from build123d import *

# Parameters (mm, degrees)
SKETCH1_W                = 45.72
SKETCH1_H                = 119.38
BOSS_EXTRUDE1_DEPTH      = 1.27
BOSS_EXTRUDE1_DEPTH_BACK = 7.636822689
SKETCH2_W                = 39.878
SKETCH2_H                = 113.538
SKETCH2_W_2              = 38.862
SKETCH2_H_2              = 112.522
BOSS_EXTRUDE2_DEPTH      = 2.54
SKETCH4_R                = 3.175
CUT_EXTRUDE1_DEPTH       = 12.446822689
SKETCH12_W               = 39.37
SKETCH12_H               = 112.522
CUT_EXTRUDE3_DEPTH       = 7.112


with BuildPart() as part:
    # Sketch1 → Boss-Extrude1 (new body, two sides)
    with BuildSketch(Plane.XY) as boss_extrude1_sk:
        with Locations((-64.545156171, 15.983606897)):
            Rectangle(SKETCH1_W, SKETCH1_H)
    extrude(amount=BOSS_EXTRUDE1_DEPTH)
    extrude(boss_extrude1_sk.sketch, amount=-BOSS_EXTRUDE1_DEPTH_BACK)

    # Sketch2 → Boss-Extrude2 (add)
    with BuildSketch(Plane.XY.offset(1.27)):
        with Locations((-64.545156171, 15.983606897)):
            Rectangle(SKETCH2_W, SKETCH2_H)
        with Locations((-64.545156171, 15.983606897)):
            Rectangle(SKETCH2_W_2, SKETCH2_H_2, mode=Mode.SUBTRACT)
    extrude(amount=BOSS_EXTRUDE2_DEPTH)

    # Sketch4 → Cut-Extrude1 (cut, through all)
    with BuildSketch(Plane(origin=(0, 0, -7.636822689), x_dir=(-1, 0, 0), z_dir=(0, 0, -1))):
        with Locations((75.500176171, 1.792626897)):
            Circle(SKETCH4_R)
    extrude(amount=-CUT_EXTRUDE1_DEPTH, mode=Mode.SUBTRACT)

    # Sketch12 → Cut-Extrude3 (cut)
    with BuildSketch(Plane.XY.offset(1.27)):
        with Locations((-64.545156171, 16.237606897)):
            Rectangle(SKETCH12_W, SKETCH12_H)
    extrude(amount=-CUT_EXTRUDE3_DEPTH, mode=Mode.SUBTRACT)


solid = part.part
Model file for the job. Use its own axes, mm. A direction names the side the tool comes from. Coordinates: 2 decimals unless noted, no trailing zeros. Order: outer loops, then holes, each group sorted by start corner. A loop starts at its lowest first (then second) coordinate and runs counter-clockwise, first axis right, second up. Notation, with made-up numbers: (29, -12.5) -> (51, -12.5) arc R22 ccw to (51, -6.5) -> close; hole circle Ø8 at (5.25, 53). An arc over 180 degrees is marked (long way). Return JSON: item names as keys, results as strings. Group by question number.
Item 1: Flat gauge pins, fed straight in: P1, Ø1.3, axis at y = 5.5, z = 3, coming from the +X side; P2, Ø12, axis at x = -71, y = 16, coming from the +Z side; P3, Ø3, axis at x = -61, z = 3, coming from the -Y side. Where does each tip first touch, or does it go through?
Item 2: Pull direction X, two halves, no side cores. Call faces 1 (the flat face through (-85, 21, 1.27)), 2 (the flat face through (-44.86, 15, -2)), 3 (the flat face through (-87.405, 15, -3)): pulls with the +X half, pulls with the -X half, needs draft (parallel to the pull), parting line crosses it, or undercut.
Item 3: Tool access for faces 4 (the flat face through (-65, 72.245, 3)), 5 (the flat face through (-65, -40.785, 3)), 6 (the flat face through (-65, 72.753, 3)), 7 (the flat face through (-84.23, 15, -2)): list every direction of +Z, -Z, +X, -X, +Y, -Y with a clear straight run to the whole face (end or side of a thin tool).
Item 4: Saw through at C-C on y = 24. Write the cut outline in (x, z), then the cut area to 3 significant figures.
Item 5: Wall check: line 1 along X through (y, z) = (-15, 3.75); line 2 along X through (y, z) = (-8, 0); line 3 along Y through (x, z) = (-74, -2.5). Give the ranges that are in metal, low to high. Write a range as [from, to].
Item 6: Saw through at A-A on z = 0. Write the cut outline in (x, y), then the cut area to 3 significant figures.
Item 7: Saw through at D-D on x = -66. Write the cut outline in (y, z), then the cut area to 3 significant figures.
Item 8: Saw through at B-B on x = -77. Write the cut outline in (y, z).
Values found:
{
 "1": {"P1": "stops at x = -44.61", "P2": "stops at z = -5.84", "P3": "stops at y = -40.79"},
 "2": {"face 1": "needs draft", "face 2": "undercut", "face 3": "pulls with the -X half"},
 "3": {"face 4": "+Z", "face 5": "+Z, +X, -X, -Y", "face 6": "+Z, +X, -X, +Y", "face 7": "none"},
 "4": {"outline": "(-87.41, -7.64) -> (-41.69, -7.64) -> (-41.69, 1.27) -> (-44.61, 1.27) -> (-44.61, 3.81) -> (-45.11, 3.81) -> (-45.11, 1.27) -> (-44.86, 1.27) -> (-44.86, -5.84) -> (-84.23, -5.84) -> (-84.23, 1.27) -> (-83.98, 1.27) -> (-83.98, 3.81) -> (-84.48, 3.81) -> (-84.48, 1.27) -> (-87.41, 1.27) -> close", "area": "130 mm2"},
 "5": {"line 1": "x = [-84.48, -83.98], [-45.11, -44.61]", "line 2": "x = [-87.41, -84.23], [-44.86, -41.69]", "line 3": "y = [-43.71, -40.02], [72.5, 75.67]"},
 "6": {"outline": "(-87.41, -43.71) -> (-41.69, -43.71) -> (-41.69, 75.67) -> (-87.41, 75.67) -> close; hole (-84.23, -40.02) -> (-44.86, -40.02) -> (-44.86, 72.5) -> (-84.23, 72.5) -> close", "area": "1,030 mm2"},
 "7": {"outline": "(-43.71, -7.64) -> (75.67, -7.64) -> (75.67, 1.27) -> (72.75, 1.27) -> (72.75, 3.81) -> (72.24, 3.81) -> (72.24, 1.27) -> (72.5, 1.27) -> (72.5, -5.84) -> (-40.02, -5.84) -> (-40.02, 1.27) -> (-40.28, 1.27) -> (-40.28, 3.81) -> (-40.79, 3.81) -> (-40.79, 1.27) -> (-43.71, 1.27) -> close", "area": "266 mm2"},
 "8": {"outline": "(-43.71, -7.64) -> (-1.01, -7.64) -> (-1.01, -5.84) -> (-40.02, -5.84) -> (-40.02, 1.27) -> (-40.28, 1.27) -> (-40.28, 3.81) -> (-40.79, 3.81) -> (-40.79, 1.27) -> (-43.71, 1.27) -> close; (4.59, -7.64) -> (75.67, -7.64) -> (75.67, 1.27) -> (72.75, 1.27) -> (72.75, 3.81) -> (72.24, 3.81) -> (72.24, 1.27) -> (72.5, 1.27) -> (72.5, -5.84) -> (4.59, -5.84) -> close"}
}
